Autodesk Inventor part; units mm, degrees
ref_plane "YZ Plane" through (0, 0, 0) normal (1, 0, 0) x (0, 1, 0)
ref_plane "XZ Plane" through (0, 0, 0) normal (0, 1, 0) x (-1, 0, 0)
ref_plane "XY Plane" through (0, 0, 0) normal (0, 0, 1) x (1, 0, 0)
sketch "Sketch1" plane through (0, 0, 0) normal (0, 0, 1) x (1, 0, 0)
  circle A0 centre (65.1069, 65.1069) radius 38.1 construction
  circle A1 centre (-56.1266, -56.1266) radius 25.4 construction
  circle A2 centre (0, 0) radius 53.975 construction
  line L0 (-38.1661, -38.1661) -> (38.1661, 38.1661) construction
  line L1 (65.1069, 65.1069) -> (-56.1266, -56.1266) construction
  line L2 (-4.3707, 6.2419) -> (-4.3707, 53.7978) construction
  line L3 (-211.1644, -81.5266) -> (654.2277, -81.5266) construction
  circle A3 centre (163.556, -24.3766) radius 57.15 construction
  circle A4 centre (65.1069, 65.1069) radius 14.2875
  circle A5 centre (-56.1266, -56.1266) radius 14.2875
  circle A6 centre (-4.3707, 6.2419) radius 57.15 construction
  circle A7 centre (-56.1266, -56.1266) radius 20.6375 construction
  circle A8 centre (65.1069, 65.1069) radius 23.8125 construction
  circle A9 centre (-73.6972, 80.6773) radius 14.2875
  line L4 (-73.6972, 80.6773) -> (65.1069, 65.1069) construction
  circle A10 centre (65.1069, 65.1069) radius 14.3256 construction
  circle A11 centre (-56.1266, -56.1266) radius 14.3256 construction
  circle A12 centre (-109.5316, 9.8231) radius 14.2875
  line L5 (-56.1266, -56.1266) -> (-109.5316, 9.8231) construction
  circle A13 centre (-109.5316, 9.8231) radius 39.7002 construction
  circle A14 centre (-73.6972, 80.6773) radius 39.7002 construction
  line L6 (17.4877, 59.0466) -> (55.9992, 43.1049)
  line L7 (-39.0193, -44.5834) -> (-51.7448, -25.7239)
  arc A15 (17.4877, 59.0466) -> (-51.7448, -25.7239) centre (-4.3707, 6.2419) ccw
  line L8 (-178.6215, 120.6011) -> (-153.6074, 116.1905) construction
  line L9 (-153.6074, 116.1905) -> (-180.0714, -33.8943) construction
  line L10 (-180.0714, -33.8943) -> (-205.0855, -29.4836) construction
  line L11 (-205.0855, -29.4836) -> (-178.6215, 120.6011) construction
  line L12 (-209.5607, -54.8639) -> (55.1963, -101.5477) construction
  line L13 (-174.1463, 145.9814) -> (158.0246, 87.4107) construction
  line L14 (-174.1463, 145.9814) -> (-209.5607, -54.8639) construction
  circle A16 centre (-138.9335, 44.7481) radius 25.4 construction
  circle A17 centre (-138.9335, 44.7481) radius 5.9531 construction
  line L15 (-84.5475, -21.0298) -> (-72.1113, -36.3871) construction
  circle A18 centre (17.7787, 70.4159) radius 9.525 construction
  line L16 (-166.1144, 118.3958) -> (-192.5784, -31.6889) construction
  line L17 (-170.5251, 93.3817) -> (-188.1678, -6.6748) construction
  circle A19 centre (-138.9335, 44.7481) radius 17.4625 construction
  circle A20 centre (-138.9335, 44.7481) radius 9.525
  circle A21 centre (-73.6972, 80.6773) radius 46.0502 construction
  line L18 (-178.6215, 120.6011) -> (-76.4165, 126.6471)
  line L19 (-61.3431, 125.0394) -> (71.4951, 88.0465)
  line L20 (-62.4968, -75.7563) -> (-205.0855, -29.4836)
  line L21 (-178.6215, 120.6011) -> (-205.0855, -29.4836)
  arc A22 (-61.3431, 125.0394) -> (-76.4165, 126.6471) centre (-73.6972, 80.6773) ccw
  arc A23 (55.9992, 43.1049) -> (71.4951, 88.0465) centre (65.1069, 65.1069) ccw
  arc A24 (-62.4968, -75.7563) -> (-39.0193, -44.5834) centre (-56.1266, -56.1266) ccw
  line L22 (-138.9335, 44.7481) -> (-128.9174, 59.0525) construction
  line L23 (-121.633, 69.4558) -> (-156.234, 20.0404) construction
  circle A25 centre (-156.234, 20.0404) radius 4.7625 construction
  line L24 (0, 0) -> (-4.3707, 6.2419) construction
  point P0 (-191.8535, 45.5588)
  point P1 (-78.3294, -28.7084)
  point P2 (-179.3464, 43.3534)
  point P3 (-179.3464, 43.3534)
  point P4 (-146.3135, 60.5745)
  point P5 (-156.3295, 46.2701)
  point P6 (-148.9496, 30.4437)
  point P7 (-131.5535, 28.9217)
  point P8 (-121.5374, 43.2261)
  point P9 (-63.3695, 121.1474)
  dimension "d7" = 50.8
  dimension "d18" = 79.4004
  dimension "d34" = 34.925
  dimension "d3" = 45
  dimension "d4" = 0
  dimension "d8" = 107.95
  dimension "d9" = 28.575
  dimension "d10" = 76.2
  dimension "d11" = 114.3
  dimension "d12" = 114.3
  dimension "d13" = 6.35
  dimension "d14" = 9.525
  dimension "d15" = 139.6746
  dimension "d16" = 28.6512
  dimension "d17" = 84.8614
  dimension "d19" = 79.4004
  dimension "d22" = 25.4
  dimension "d23" = 152.4
  dimension "d26" = 203.9436
  dimension "d27" = 50.8
  dimension "d28" = 11.9062
  dimension "d29" = 51
  dimension "d30" = 171.45
  dimension "d31" = 10
  dimension "d32" = 19.05
  dimension "d33" = 101.6
  dimension "d35" = 19.05
  dimension "d36" = 6.35
  dimension "d37" = 34.925
  dimension "d40" = 360
  dimension "d43" = 25
  dimension "d44" = 9.525
  dimension "d55" = 80
  dimension "d56" = 7.62
extrude "Extrusion1" add sketch "Sketch1" along normal blind 6.35
hole "Hole1" at (-78.3294, -28.7084, 0) at (17.7787, 70.4159, 0) at (-170.5251, 93.3817, 0) at (-179.3464, 43.3534, 0) at (-188.1678, -6.6748, 0) at (-128.9174, 59.0525, 0) at (-146.3135, 60.5745, 0) at (-156.3295, 46.2701, 0) at (-148.9496, 30.4437, 0) at (-131.5535, 28.9217, 0) at (-121.5374, 43.2261, 0) at (-121.633, 69.4558, 0) at (-156.234, 20.0404, 0) direction (0, 0, 1) diameter 5.1054 end through all
properties part number "GP7-001" material "Polycarbonate, Smoke"
Can you work these out from the model? Positions are in its coordinate system, mm. A direction names the side the tool comes from. Round coordinates to 2 decimals unless told otherwise and drop trailing zeros. Loops run counter-clockwise (first coordinate to the right, second up) from the corner with the lowest first, then second, coordinate; pieces in that order, holes last. Notation, with made-up numbers: (11.5, -35.5) -> (41.5, -35.5) arc R15 cw to (41.5, -21.5) -> close; hole circle Ø6 at (55.5, 46). An arc over 180 degrees is marked (long way). One line per item, written item: value. Start each with the question number.
1. If we section it at C-C, the plane x = -7: Write out the boundary of the cut face in (y, z).
2. If I drill on probe 1 along Y at (x, z) = (-158, 5.5); probe 2 along X at (y, z) = (29, 3.25) (3 decimals); probe 3 along Y at (x, z) = (-81.5, 0.5), over which ranges is the centre line in solid material (lowest first)?
3. If we section it at B-B, the plane y = -21.5: Write out the boundary of the cut face in (x, z), then the cut area to 3 significant figures.
4. If we mould it in two halves opening along X, with no side actions, what happens to faces 4 (the flat face through (-128.234, 123.582, 3.131)), 5 (the cylindrical face through (71.7, 77.78, 3.13)), 6 (the flat face through (-93, 49, 6.35)), 7 (the cylindrical face through (-95.904, 5.532, 3.131))? For each: pulls with the +X half, pulls with the -X half, needs draft (parallel to the pull), parting line crosses it, or undercut.
5. For faces 1 (the flat face through (-45.29, -35.29, 3.13)), 2 (the flat face through (4.15, 106.8, 3.13)), 3 (the flat face through (36.47, 51.19, 3.13)), which set-ups out of +Z, -Z, +X, -X, +Y, -Y let a thin tool reach every point of the face, with its end or its side?
6. For pin 1 (17 mm diameter, centred on x = 65.11, y = 65.11, fed in from -Z); pin 2 (1 mm diameter, centred on x = -57.5, z = 5, fed in from -Y); pin 3 (2 mm diameter, centred on x = 12, z = 4.5, fed in from -Y); pin 4 (1 mm diameter, centred on x = 16, z = 5.5, fed in from +Y), each with a flat end and sliding along its axis, tell me the tip position at first contact or that it passes through.
7. If we section it at A-A, the plane z = 1: Give the number of separate pieces and of enclosed holes in the cut face, then the cut area to 3 significant figures.
Calculated:
1. outline: (63.33, 0) -> (109.91, 0) -> (109.91, 6.35) -> (63.33, 6.35) -> close
2. probe 1: y = -44.76 to 18.2, 21.88 to 44.34, 48.2 to 121.82
2. probe 2: x = -194.773 to -151.055, -146.844 to -134.105, -129.002 to -56.794
2. probe 3: y = -69.59 to 68.71, 92.65 to 126.35
3. outline: (-203.68, 0) -> (-54.34, 0) -> (-54.34, 6.35) -> (-203.68, 6.35) -> close
3. area: 948 mm²
4. face 4: pulls with the -X half
4. face 5: undercut
4. face 6: needs draft
4. face 7: undercut
5. face 1: +Z, -Z, +X
5. face 2: +Z, -Z, +X, +Y
5. face 3: +Z, -Z, -Y
6. pin 1: passes through
6. pin 2: stops at y = -76.75
6. pin 3: stops at y = 60.69
6. pin 4: stops at y = 103.64
7. separate pieces: 1
7. enclosed holes: 18
7. area: 29,200 mm²
